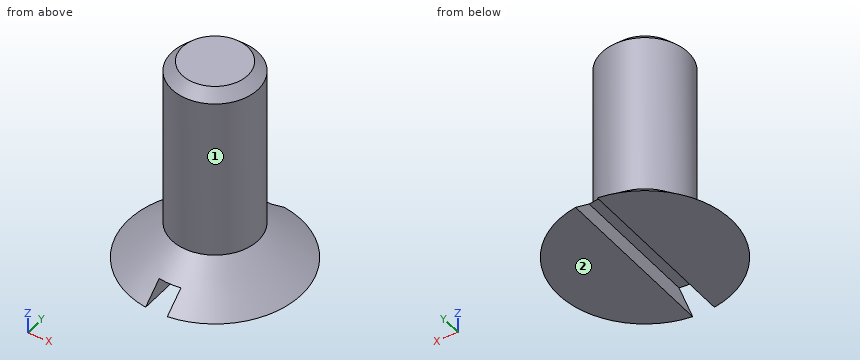
```python
from build123d import *

# Parameters (mm, degrees)
SKETCH6_W          = 1.6002
SKETCH6_H          = 14.426568413
CUT_EXTRUDE2_DEPTH = 1.27


with BuildPart() as part:
    # Sketch5 → Revolve2 (revolve)
    with BuildSketch(Plane(origin=(0, 0, 0), x_dir=(1, 0, 0), z_dir=(0, 1, 0))):
        Polygon((0, 14.732), (0, -0.762), (2.413, -0.762), (3.175, 0), (3.175, 11.938), (6.3754, 14.732), align=None)
    revolve(axis=Axis((0, 0, 0), (0, 0, 1)))

    # Sketch6 → Cut-Extrude2 (cut)
    with BuildSketch(Plane(origin=(0, 0, -14.732), x_dir=(-1, 0, 0), z_dir=(0, 0, -1))):
        with Locations((0, 0.400071831)):
            Rectangle(SKETCH6_W, SKETCH6_H)
    extrude(amount=-CUT_EXTRUDE2_DEPTH, mode=Mode.SUBTRACT)


solid = part.part
```
CAD build for the part. Positions are in the model's coordinates, mm. Face numbers are marked on the shaded views. A direction names the side the tool comes from. Round coordinates to 2 decimals unless told otherwise and drop trailing zeros. Order: outer loops, then holes, each group sorted by start corner. A loop starts at its lowest first (then second) coordinate and runs counter-clockwise, first axis right, second up.
Q1. Slice it at C-C (z = -7.5). Write the cut outline in (x, y) (3 decimals), and give its area (3 significant figures).
Q2. Drop flat-ended pins along their axis: pin 1 (1.5 mm diameter, centred on y = -5, z = -2, fed in from +X); pin 2 (1 mm diameter, centred on y = 1.5, z = -14, fed in from +X); pin 3 (0.6 mm diameter, centred on y = 0.5, z = -14.5, fed in from -X); pin 4 (3 mm diameter, centred on y = -1, z = -11.5, fed in from -X). Give the stop position or say it passes through.
Q3. Wall check: L1, parallel to Z at x = -0.25, y = 0.25; L2, parallel to Z at x = -2, y = 4.5; L3, parallel to Y at x = 1.75, z = -14. Give the ranges that are in metal, low to high.
Q4. Slice it at B-B (x = 0). Write the cut outline in (y, z) (3 decimals), and give its area (3 significant figures).
Q5. Slice it at A-A (y = 0). Write the cut outline in (x, z) (3 decimals).
Q6. Which spindle directions (+Z, -Z, +X, -X, +Y, -Y) get a long thin tool onto all of the face, cutting with end or side? Do the marked faces 1 and 2. Say none if no direction does.
Results below:
1. outline: circle Ø6.35 at (0, 0)
1. area: 31.7 mm2
2. pin 1: passes through
2. pin 2: stops at x = 5.94
2. pin 3: stops at x = -6.37
2. pin 4: stops at x = -4.3
3. L1: z = -13.46 to 0.76
3. L2: z = -14.73 to -13.47
3. L3: y = -5.25 to 5.25
4. outline: (-4.921, -13.462) - (4.921, -13.462) - (3.175, -11.938) - (3.175, 0) - (2.413, 0.762) - (-2.413, 0.762) - (-3.175, 0) - (-3.175, -11.938) - close
4. area: 92.4 mm2
5. outline: (-6.375, -14.732) - (-0.8, -14.732) - (-0.8, -13.462) - (0.8, -13.462) - (0.8, -14.732) - (6.375, -14.732) - (3.175, -11.938) - (3.175, 0) - (2.413, 0.762) - (-2.413, 0.762) - (-3.175, 0) - (-3.175, -11.938) - close
6. face 1: +Z
6. face 2: -Z, +X, -X, +Y, -Y
